Geometry: final body of the model. Coordinates: model frame, mm. A direction names the side the tool comes from. Give positions to 0.01 mm unless a question says otherwise; leave off trailing zeros. Loops run counter-clockwise (first coordinate to the right, second up) from the corner with the lowest first, then second, coordinate; pieces in that order, holes last.
1. Draft query along X for faces 1 (the face through (-14.524, -45.982, 1.479)), 2 (the face through (-17, 60, 3)), 3 (the face through (-11.908, -44, 1)). Return one class per face: +X half, -X half, draft (parallel to the pull), parting line (faces both ways), or undercut.
2. Section C-C, the plane y = -35. Output: boundary loops of the cut face in (x, z), then the cut area to 3 significant figures.
3. Section A-A, the plane z = 82.5. Output: boundary loops of the cut face in (x, y).
4. First-contact query: P1, Ø1.5, axis at x = -10.5, z = 93.5, coming from the -Y side; P2, Ø10, axis at x = -13.5, z = 74, coming from the +Y side; P3, Ø10, axis at x = -34, y = 18, coming from the -Z side. Flat tips, straight axial feed; report the tip coordinate or a pass-through.
5. Access query for faces 4 (the face through (-18, 24.897, 94)), 5 (the face through (15, 14, 6)), 6 (the face through (15, 14, 4)). Directions: +Z, -Z, +X, -X, +Y, -Y. A direction counts if a zero-diameter tool reaches every point of the face in a straight line with its end or side. Return the directions, or none.
6. Section D-D, the plane y = -2.5. Output: boundary loops of the cut face in (x, z), then the cut area to 3 significant figures.
7. Section B-B, the plane x = 1. State how many separate pieces and enclosed holes the cut face has, then the cut area to 3 significant figures.
8. Material intervals for line 1 along X through (y, z) = (-10, 55); line 2 along Y through (x, z) = (-22, 54.5); line 3 along X through (y, z) = (36, 5.5), sorted ascending.
from build123d import *

# Parameters (mm, degrees)
ESBO_O1_W                = 72
ESBO_O1_H                = 100
ESBO_O1_W_2              = 66
ESBO_O1_H_2              = 94
RESSALTO_EXTRUS_O1_DEPTH = 92
ESBO_O2_W                = 72
ESBO_O2_H                = 100
RESSALTO_EXTRUS_O2_DEPTH = 3
RESSALTO_EXTRUS_O3_START = -95
ESBO_O3_R                = 2.5
RESSALTO_EXTRUS_O3_DEPTH = 3
CORTE_EXTRUS_O1_DEPTH    = 3
RESSALTO_EXTRUS_O4_START = 4
ESBO_O5_W                = 4
ESBO_O5_H                = 84
RESSALTO_EXTRUS_O4_DEPTH = 2


with BuildPart() as part:
    # Esboço1 → Ressalto-extrusão1 (new body)
    with BuildSketch(Plane.XY):
        with Locations((-15.908396947, 8.267175573)):
            Rectangle(ESBO_O1_W, ESBO_O1_H)
        with Locations((-15.908396947, 8.267175573)):
            Rectangle(ESBO_O1_W_2, ESBO_O1_H_2, mode=Mode.SUBTRACT)
    extrude(amount=RESSALTO_EXTRUS_O1_DEPTH)

    # Esboço2 → Ressalto-extrusão2 (add)
    with BuildSketch(Plane.XY.offset(92)):
        with Locations((-15.908396947, 8.267175573)):
            Rectangle(ESBO_O2_W, ESBO_O2_H)
    extrude(amount=RESSALTO_EXTRUS_O2_DEPTH)

    # Esboço3 → Ressalto-extrusão3 (add)
    # profile 1 of 2: a face of its own
    with BuildSketch(Plane.XY.offset(95).offset(RESSALTO_EXTRUS_O3_START)):
        with BuildLine():
            Line((-21.908396947, 58.267175573), (-21.908396947, 63.267175573))
            ThreePointArc((-21.908396947, 63.267175573), (-16.908396947, 68.267175573), (-11.908396947, 63.267175573))
            Line((-11.908396947, 63.267175573), (-11.908396947, 58.267175573))
            Line((-11.908396947, 58.267175573), (-21.908396947, 58.267175573))
        make_face()
        with Locations((-16.908396947, 63.267175573)):
            Circle(ESBO_O3_R, mode=Mode.SUBTRACT)
    # profile 2 of 2: a face of its own
    with BuildSketch(Plane.XY.offset(95).offset(RESSALTO_EXTRUS_O3_START)):
        with BuildLine():
            Line((-11.908396947, -46.732824427), (-11.908396947, -41.732824427))
            Line((-11.908396947, -41.732824427), (-21.908396947, -41.732824427))
            Line((-21.908396947, -41.732824427), (-21.908396947, -46.732824427))
            ThreePointArc((-21.908396947, -46.732824427), (-16.908396947, -51.732824427), (-11.908396947, -46.732824427))
        make_face()
        with Locations((-16.908396947, -46.732824427)):
            Circle(ESBO_O3_R, mode=Mode.SUBTRACT)
    extrude(amount=RESSALTO_EXTRUS_O3_DEPTH)

    # Esboço4 → Corte-extrusão1 (cut)
    with BuildSketch(Plane.XY.offset(95)):
        with BuildLine():
            Line((-42.438758468, 27.697077942), (7.561241532, 27.697077942))
            ThreePointArc((7.561241532, 27.697077942), (7.961241532, 27.297077942), (7.561241532, 26.897077942))
            Line((7.561241532, 26.897077942), (-42.438758468, 26.897077942))
            ThreePointArc((-42.438758468, 26.897077942), (-42.838758468, 27.297077942), (-42.438758468, 27.697077942))
        make_face()
        with BuildLine():
            Line((-42.438758468, 24.897077942), (7.561241532, 24.897077942))
            ThreePointArc((7.561241532, 24.897077942), (7.961241532, 24.497077942), (7.561241532, 24.097077942))
            Line((7.561241532, 24.097077942), (-42.438758468, 24.097077942))
            ThreePointArc((-42.438758468, 24.097077942), (-42.838758468, 24.497077942), (-42.438758468, 24.897077942))
        make_face()
        with BuildLine():
            Line((-42.438758468, 22.097077942), (7.705579096, 22.097077942))
            ThreePointArc((7.705579096, 22.097077942), (8.105579096, 21.697077942), (7.705579096, 21.297077942))
            Line((7.705579096, 21.297077942), (-42.438758468, 21.297077942))
            ThreePointArc((-42.438758468, 21.297077942), (-42.838758468, 21.697077942), (-42.438758468, 22.097077942))
        make_face()
        with BuildLine():
            Line((-42.438758468, 19.297077942), (7.705579096, 19.297077942))
            ThreePointArc((7.705579096, 19.297077942), (8.105579096, 18.897077942), (7.705579096, 18.497077942))
            Line((7.705579096, 18.497077942), (-42.438758468, 18.497077942))
            ThreePointArc((-42.438758468, 18.497077942), (-42.838758468, 18.897077942), (-42.438758468, 19.297077942))
        make_face()
        with BuildLine():
            Line((-42.438758468, 16.497077942), (7.561241532, 16.497077942))
            ThreePointArc((7.561241532, 16.497077942), (7.961241532, 16.097077942), (7.561241532, 15.697077942))
            Line((7.561241532, 15.697077942), (-42.438758468, 15.697077942))
            ThreePointArc((-42.438758468, 15.697077942), (-42.838758468, 16.097077942), (-42.438758468, 16.497077942))
        make_face()
        with BuildLine():
            Line((-42.438758468, 13.697077942), (7.561241532, 13.697077942))
            ThreePointArc((7.561241532, 13.697077942), (7.961241532, 13.297077942), (7.561241532, 12.897077942))
            Line((7.561241532, 12.897077942), (-42.438758468, 12.897077942))
            ThreePointArc((-42.438758468, 12.897077942), (-42.838758468, 13.297077942), (-42.438758468, 13.697077942))
        make_face()
        with BuildLine():
            Line((-42.438758468, 10.897077942), (7.705579175, 10.897077942))
            ThreePointArc((7.705579175, 10.897077942), (8.105579175, 10.497077942), (7.705579175, 10.097077942))
            Line((7.705579175, 10.097077942), (-42.438758468, 10.097077942))
            ThreePointArc((-42.438758468, 10.097077942), (-42.838758468, 10.497077942), (-42.438758468, 10.897077942))
        make_face()
        with BuildLine():
            Line((-42.438758468, 8.097077942), (7.705579175, 8.097077942))
            ThreePointArc((7.705579175, 8.097077942), (8.105579175, 7.697077942), (7.705579175, 7.297077942))
            Line((7.705579175, 7.297077942), (-42.438758468, 7.297077942))
            ThreePointArc((-42.438758468, 7.297077942), (-42.838758468, 7.697077942), (-42.438758468, 8.097077942))
        make_face()
    extrude(amount=-CORTE_EXTRUS_O1_DEPTH, mode=Mode.SUBTRACT)

    # Esboço5 → Ressalto-extrusão4 (add)
    with BuildSketch(Plane.XY.offset(RESSALTO_EXTRUS_O4_START)):
        with Locations((-46.908396947, 13.267175573)):
            Rectangle(ESBO_O5_W, ESBO_O5_H)
        with Locations((15.091603053, 13.267175573)):
            Rectangle(ESBO_O5_W, ESBO_O5_H)
    extrude(amount=RESSALTO_EXTRUS_O4_DEPTH)


solid = part.part
Answers below:
1. face 1: undercut
1. face 2: draft
1. face 3: +X half
2. outline: (-51.91, 0) - (-48.91, 0) - (-48.91, 92) - (17.09, 92) - (17.09, 0) - (20.09, 0) - (20.09, 95) - (-51.91, 95) - close
2. area: 768 mm2
3. outline: (-51.91, -41.73) - (20.09, -41.73) - (20.09, 58.27) - (-51.91, 58.27) - close; hole (-48.91, -38.73) - (17.09, -38.73) - (17.09, 55.27) - (-48.91, 55.27) - close
4. P1: stops at y = -41.73
4. P2: stops at y = 58.27
4. P3: stops at z = 92
5. face 4: +Z, -Z
5. face 5: none
5. face 6: -Z
6. outline: (-51.91, 0) - (-48.91, 0) - (-48.91, 4) - (-44.91, 4) - (-44.91, 6) - (-48.91, 6) - (-48.91, 92) - (17.09, 92) - (17.09, 6) - (13.09, 6) - (13.09, 4) - (17.09, 4) - (17.09, 0) - (20.09, 0) - (20.09, 95) - (-51.91, 95) - close
6. area: 784 mm2
7. separate pieces: 9
7. enclosed holes: 0
7. area: 833 mm2
8. line 1: x = -51.91 to -48.91, 17.09 to 20.09
8. line 2: y = -41.73 to -38.73, 55.27 to 58.27
8. line 3: x = -51.91 to -44.91, 13.09 to 20.09
